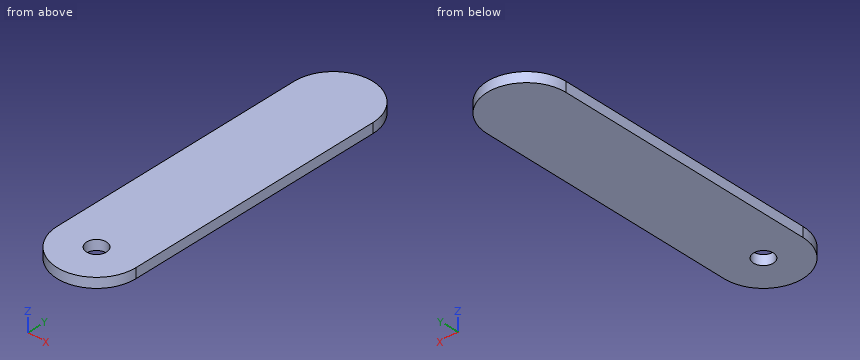
Autodesk Inventor part; units mm, degrees
ref_plane "YZ Plane" through (0, 0, 0) normal (1, 0, 0) x (0, 1, 0)
ref_plane "XZ Plane" through (0, 0, 0) normal (0, 1, 0) x (-1, 0, 0)
ref_plane "XY Plane" through (0, 0, 0) normal (0, 0, 1) x (1, 0, 0)
ref_plane "Work Plane1" through (0, 0, 0) normal (0, 0, 1) x (1, 0, 0)
sketch "Sketch1" plane through (0, 0, 0) normal (0, 0, 1) x (1, 0, 0)
  circle A0 centre (0, 107.5) radius 10
  circle A1 centre (0, 107.5) radius 5
  line L0 (20, 237.5) -> (-20, 237.5)
  line L1 (-20, 237.5) -> (-20, 87.5)
  line L2 (-20, 87.5) -> (20, 87.5)
  line L3 (20, 87.5) -> (20, 237.5)
  circle A2 centre (0, 107.5) radius 20
  circle A3 centre (0, 237.5) radius 20
  point P0 (0, 0)
  point P1 (-20, 107.5)
  point P2 (20, 107.5)
  dimension "d0" = 40
  dimension "d1" = 150
  dimension "d2" = 20
  dimension "d4" = 20
  dimension "d5" = 40
  dimension "d6" = 130
extrude "Extrusion1" add sketch "Sketch1" along normal blind 5 contours A0 | A3 L0 | L0 A3 | L3 A2 L1 A3 | A2
properties part number "Link3base"
Geometry check sheet. Reference: the model listing, model coordinates, mm. Coordinates: 2 decimals unless noted, no trailing zeros. Order: outer loops, then holes, each group sorted by start corner. A loop starts at its lowest first (then second) coordinate and runs counter-clockwise, first axis right, second up. Notation, with made-up numbers: (54.5, -36) - (62.5, -36) arc R18 cw to (62.5, -10) - close; hole circle Ø11 at (-29.75, -14). An arc over 180 degrees is marked (long way). Answer as a JSON object with one key per item and string values. Group by question number.
Item 1: Scan lines: probe 1 along Y at (x, z) = (0, 3.7); probe 2 along Y at (x, z) = (3, 4.6); probe 3 along Y at (x, z) = (10.5, 4.25). Record each from-to range of solid material in increasing order.
Item 2: Sectioned sample at D-D, the plane x = 10. Record the cut outline in (y, z), and give its area (3 significant figures).
Item 3: Sectioned sample at A-A, the plane x = 0. Record the cut outline in (y, z).
Item 4: Sectioned sample at C-C, the plane x = -15. Record the cut outline in (y, z), and give its area (3 significant figures).
Item 5: Sectioned sample at B-B, the plane z = 3.65. Record the cut outline in (x, y), and give its area (3 significant figures).
Resolved:
{
 "1": {"probe 1": "87.5 to 102.5, 112.5 to 257.5", "probe 2": "87.73 to 103.5, 111.5 to 257.27", "probe 3": "90.48 to 254.52"},
 "2": {"outline": "(90.18, 0) - (254.82, 0) - (254.82, 5) - (90.18, 5) - close", "area": "823 mm^2"},
 "3": {"outline": "(87.5, 0) - (102.5, 0) - (102.5, 5) - (87.5, 5) - close; (112.5, 0) - (257.5, 0) - (257.5, 5) - (112.5, 5) - close"},
 "4": {"outline": "(94.27, 0) - (250.73, 0) - (250.73, 5) - (94.27, 5) - close", "area": "782 mm^2"},
 "5": {"outline": "(-20, 107.5) arc R20 ccw to (20, 107.5) - (20, 237.5) arc R20 ccw to (-20, 237.5) - close; hole circle Ø10 at (0, 107.5)", "area": "6,380 mm^2"}
}
